Work out the finished part from the listing and answer in its coordinate system (mm). Coordinates: 2 decimals unless noted, no trailing zeros. Write each loop counter-clockwise with the first axis right and the second up, starting at its lowest first coordinate (ties: lowest second). Pieces come first, ordered by that corner, then holes. Notation, with made-up numbers: (-40, -1) - (-23, -1) arc R15 ccw to (-23, 8) - close; hole circle Ø10 at (34, 11.5). An arc over 180 degrees is marked (long way). Use one line per item in the form item = value. Start each with the question number.
Item 1: Consider probe 1 along Y at (x, z) = (-75.5, 4.5); probe 2 along X at (y, z) = (-1, 4); probe 3 along Y at (x, z) = (-41, 5). Determine where each line is inside the solid, lowest interval first.
Item 2: A cutting plane is placed at B-B (z = 3.25). Write down the section's boundary in (x, y).
Item 3: A cutting plane is placed at A-A (y = 6.5). Write down the section's boundary in (x, z), then the cut area to 3 significant figures.
Item 4: Given pin 1 (2 mm diameter, centred on y = -8, z = 2, fed in from +X), flat-ended and moving along its own axis, determine where the tip first touches the part or whether it passes through.
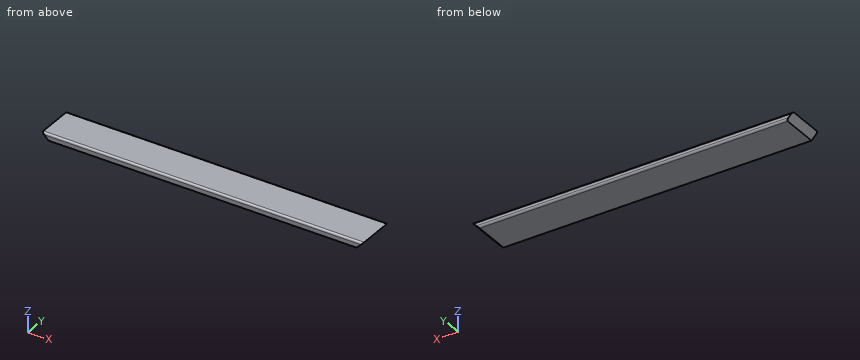
from build123d import *

# Parameters (mm, degrees)
BOSS_EXTRUDE1_DEPTH = 19.05
FILLET1_R           = 2


with BuildPart() as part:
    # Sketch1 → Boss-Extrude1 (new body, symmetric)
    with BuildSketch(Plane(origin=(0, 0, 0), x_dir=(1, 0, 0), z_dir=(0, 1, 0))):
        Polygon((-153, 0), (153, 0), (159.35, -6.35), (-159.35, -6.35), align=None)
    extrude(amount=BOSS_EXTRUDE1_DEPTH, both=True)

    # Fillet1
    fillet1_edges = [part.edges().sort_by_distance(p)[0] for p in [
        (0, 19.05, 0),
        (0, -19.05, 6.35),
        (0, 19.05, 6.35),
    ]]
    fillet(fillet1_edges, radius=FILLET1_R)


solid = part.part
Answer:
q1.probe_1 = -19.04 to 19.04
q1.probe_2 = -157 to 157
q1.probe_3 = -18.94 to 18.94
q2.outline = (-156.25, -19.05) - (156.25, -19.05) - (156.25, 19.05) - (-156.25, 19.05) - close
q3.outline = (-159.35, 6.35) - (-153, 0) - (153, 0) - (159.35, 6.35) - close
q3.area = 1,980 mm²
q4.pin_1 = 156
